```python
from build123d import *

# Parameters (mm, degrees)
PAD_DEPTH       = 5
POCKET_DEPTH    = 2
SKETCH002_R     = 1.7
POCKET001_DEPTH = 4.001


with BuildPart() as part:
    # Sketch → Pad (new body, symmetric)
    with BuildSketch(Plane.XY):
        with BuildLine():
            ThreePointArc((2, -7.745967), (8, 0), (2, 7.745967))
            Line((2, 7.745967), (2, -7.745967))
        make_face()
    extrude(amount=PAD_DEPTH, both=True)

    # Sketch001 → Pocket (cut)
    with BuildSketch(Plane(origin=(2, 0, 0), x_dir=(0, -1, 0), z_dir=(-1, 0, 0))):
        Polygon((2.8, -1.616581), (2.8, 1.616581), (0, 3.233162), (-2.8, 1.616581), (-2.8, -1.616581), (0, -3.233162), align=None)
    extrude(amount=-POCKET_DEPTH, mode=Mode.SUBTRACT)

    # Sketch002 → Pocket001 (cut, through all)
    with BuildSketch(Plane(origin=(4, 0, 0), x_dir=(0, -1, 0), z_dir=(-1, 0, 0))):
        Circle(SKETCH002_R)
    extrude(amount=-POCKET001_DEPTH, mode=Mode.SUBTRACT)


solid = part.part
```
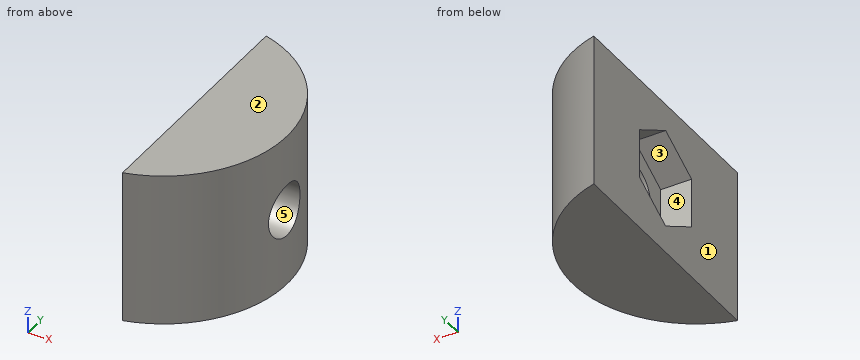
Read the model definition and answer for the solid it produces. Units are mm, in the model's axes. Face numbers are marked on the shaded views. A direction names the side the tool comes from. Coordinates: 2 decimals unless noted, no trailing zeros. Loops run counter-clockwise (first coordinate to the right, second up) from the corner with the lowest first, then second, coordinate; pieces in that order, holes last. Notation, with made-up numbers: (-2.75, 5.5) - (3.25, 5.5) arc R7 cw to (3.25, 11.5) - close; hole circle Ø1 at (18.5, 28). An arc over 180 degrees is marked (long way). Answer in a Markdown table with one row per item.
1. Find section D-D, the plane z = 0. Write down the section's boundary in (x, y).
Conclusion:
| item | result |
|---|---|
| outline | (2, -7.75) arc R8 ccw to (7.82, -1.7) - (4, -1.7) - (4, -2.8) - (2, -2.8) - close; (2, 2.8) - (4, 2.8) - (4, 1.7) - (7.82, 1.7) arc R8 ccw to (2, 7.75) - close |
2. Find section C-C, the plane x = 6.25. Write down the section's boundary in (y, z), then the cut area to 3 significant figures.
Conclusion:
| item | result |
|---|---|
| outline | (-4.99, -5) - (4.99, -5) - (4.99, 5) - (-4.99, 5) - close; hole circle Ø3.4 at (0, 0) |
| area | 90.8 mm² |
3. Straight lines are drawn through the part: line 1 (Z direction, x = 6.85, y = 0); line 2 (X direction, y = -0.25, z = 4.5); line 3 (Y direction, x = 5.9, z = 0). For each, find the intervals that lie inside material, in ascending order.
Conclusion:
| item | result |
|---|---|
| line 1 | z = -5 to -1.7, 1.7 to 5 |
| line 2 | x = 2 to 8 |
| line 3 | y = -5.4 to -1.7, 1.7 to 5.4 |
4. Find section B-B, the plane y = -1.5. Write down the section's boundary in (x, z), then the cut area to 3 significant figures.
Conclusion:
| item | result |
|---|---|
| outline | (2, -5) - (7.86, -5) - (7.86, -0.8) - (4, -0.8) - (4, -2.37) - (2, -2.37) - close; (2, 2.37) - (4, 2.37) - (4, 0.8) - (7.86, 0.8) - (7.86, 5) - (2, 5) - close |
| area | 42.9 mm² |
5. Which of the six approach directions +Z, -Z, +X, -X, +Y, -Y give full straight-line access (tool end or side, diameter ignored) to the marked faces 4 and 5?
Conclusion:
| item | result |
|---|---|
| face 4 | -X |
| face 5 | +X, -X |
6. Find section A-A, the plane z = 1.25. Write down the section's boundary in (x, y).
Conclusion:
| item | result |
|---|---|
| outline | (2, -7.75) arc R8 ccw to (7.92, -1.15) - (4, -1.15) - (4, -2.8) - (2, -2.8) - close; (2, 2.8) - (4, 2.8) - (4, 1.15) - (7.92, 1.15) arc R8 ccw to (2, 7.75) - close |
7. Determine the mould class of the marked faces 1, 2 and 3 for opening direction Z: +Z half, -Z half, draft (parallel to the pull), parting line (faces both ways), or undercut.
Conclusion:
| item | result |
|---|---|
| face 1 | draft |
| face 2 | +Z half |
| face 3 | undercut |
8. Given pin 1 (2.5 mm diameter, centred on y = 0, z = 0, fed in from +X); pin 2 (2 mm diameter, centred on x = 3.5, z = 0, fed in from +Y); pin 3 (2 mm diameter, centred on y = 5.5, z = -0.5, fed in from +X); pin 4 (3 mm diameter, centred on x = 4.5, z = 2, fed in from +Y), each flat-ended and moving along its own axis, determine where each tip first touches the part or whether it passes through.
Conclusion:
| item | result |
|---|---|
| pin 1 | passes through |
| pin 2 | stops at y = 7.6 |
| pin 3 | stops at x = 6.61 |
| pin 4 | stops at y = 7.42 |
